For this review, take the finished solid that the model builds, in its own axes (mm). Face numbers are marked on the shaded views. A direction names the side the tool comes from. Give positions to 0.01 mm unless a question says otherwise; leave off trailing zeros. Order: outer loops, then holes, each group sorted by start corner. A loop starts at its lowest first (then second) coordinate and runs counter-clockwise, first axis right, second up. Notation, with made-up numbers: M 7,46 L 17,46 A9 cw 17,54 Z; hole C 1,69 d5. An arc over 180 degrees is marked long. Answer as CSV lines item,"result". Start each with the question number.
1. Clearance check with flat-ended pins moving along their axes: P1, Ø4, axis at x = -19.69, z = 24.25, coming from the -Y side; P2, Ø5, axis at x = -19.5, z = 26, coming from the +Y side; P3, Ø4.5, axis at x = -19.69, z = 9.25, coming from the +Y side. State where each tip first meets the part, or that it passes through.
2. We need section C-C, the plane y = -9. Give the boundary of the cut face in (x, z), and give its area (3 significant figures).
3. Machinability: for the marked faces 1, 2 and 3, which of the approach directions +Z, -Z, +X, -X, +Y, -Y give a long, thin tool a straight path to every point of the face, cutting with its end or side? Answer none if there is none.
4. Mouldability with a two-part tool opening along Z and no side actions: class the marked faces 4, 5, 6 and 7 as pulls with the +Z half, pulls with the -Z half, needs draft (parallel to the pull), parting line crosses it, or undercut.
5. We need section B-B, the plane x = -3. Give the boundary of the cut face in (y, z), and give its area (3 significant figures).
6. We need section D-D, the plane z = 17. Give the boundary of the cut face in (x, y), and give its area (3 significant figures).
7. For line 1 along X through (y, z) = (15, 9.25); line 2 along X through (y, z) = (8, -24); line 3 along Y through (x, z) = (0, -1), list the stretches that pass through material, from the lowest coordinate up.
8. We need section A-A, the plane y = 6.5. Give the boundary of the cut face in (x, z), and give its area (3 significant figures).
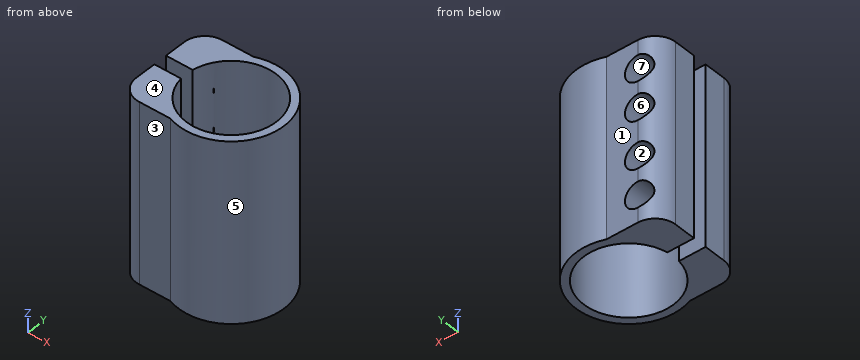
from build123d import *

# Parameters (mm, degrees)
F1_DEPTH       = 35
F3_D           = 5
F3_DEPTH       = 12
F3_START       = 1.7550021
F3_CBORE_D     = 10
F3_CBORE_DEPTH = 8
F3_TIP         = 1.5021515476


with BuildPart() as f1:
    # F0 (on Top) → F1 (new body, symmetric)
    with BuildSketch(Plane.XY):
        with BuildLine():
            ThreePointArc((-17.2933548246, 2.6813949562), (17.5, 0), (-17.2933548246, -2.6813949562))
            Line((-17.2933548246, -2.6813949562), (-27.6933548246, -2.6813949562))
            Line((-27.6933548246, -2.6813949562), (-27.6933548246, -11.0813949562))
            ThreePointArc((-27.6933548246, -11.0813949562), (-25.3502090741, -16.7382492056), (-19.6933548246, -19.0813949562))
            Line((-19.6933548246, -19.0813949562), (-7.4933548246, -19.0813949562))
            ThreePointArc((-7.4933548246, -19.0813949562), (20.5, 0), (-7.4933548246, 19.0813949562))
            Line((-7.4933548246, 19.0813949562), (-19.6933548246, 19.0813949562))
            ThreePointArc((-19.6933548246, 19.0813949562), (-25.3502090741, 16.7382492056), (-27.6933548246, 11.0813949562))
            Line((-27.6933548246, 11.0813949562), (-27.6933548246, 2.6813949562))
            Line((-27.6933548246, 2.6813949562), (-17.2933548246, 2.6813949562))
        make_face()
    extrude(amount=F1_DEPTH, both=True)

    # F3
    # its depths count from where the whole tool has entered the part; down to there all is cleared
    with Locations(Plane(origin=(0, 19.0813949562, 0), x_dir=(-1, 0, 0), z_dir=(0, 1, 0)).offset(-F3_START)):
        with Locations((19.6933548246, 24.25), (19.6933548246, 9.25), (19.6933548246, -9.25), (19.6933548246, -24.25)):
            CounterBoreHole(F3_D / 2, F3_CBORE_D / 2, F3_CBORE_DEPTH, depth=F3_DEPTH)
            with Locations((0, 0, -(F3_DEPTH + F3_TIP / 2))):  # 118° drill point
                Cone(0, F3_D / 2, F3_TIP, mode=Mode.SUBTRACT)


solid = f1.part
Result set:
1,P1,"y = -19.08"
1,P2,"y = 9.33"
1,P3,"y = 5.18"
2,outline,"M -27.69,-35 L -15.01,-35 L -15.01,35 L -27.69,35 Z; M 15.01,-35 L 18.42,-35 L 18.42,35 L 15.01,35 Z"
2,area,"1,130 mm2"
3,face 1,"+Z, -Z, -X, +Y"
3,face 2,"+Y"
3,face 3,"+Z, -Z, -X, -Y"
4,face 4,"pulls with the +Z half"
4,face 5,"needs draft"
4,face 6,"undercut"
4,face 7,"undercut"
5,outline,"M -20.28,-35 L -17.24,-35 L -17.24,35 L -20.28,35 Z; M 17.24,-35 L 20.28,-35 L 20.28,35 L 17.24,35 Z"
5,area,"425 mm2"
6,outline,"M -27.69,-11.08 A8 ccw -19.69,-19.08 L -7.49,-19.08 A20.5 ccw long -7.49,19.08 L -19.69,19.08 A8 ccw -27.69,11.08 L -27.69,2.68 L -17.29,2.68 A17.5 cw long -17.29,-2.68 L -27.69,-2.68 Z"
6,area,"687 mm2"
7,line 1,"-26.67 to -24.69, -14.69 to -9.01, 9.01 to 13.97"
7,line 2,"-27.69 to -22.18, -17.21 to -15.56, 15.56 to 18.87"
7,line 3,"-20.5 to -17.5, 17.5 to 20.5"
8,outline,"M -27.69,-35 L -16.25,-35 L -16.25,35 L -27.69,35 Z; M 16.25,-35 L 19.44,-35 L 19.44,35 L 16.25,35 Z; hole C -19.69,-24.25 d5; hole C -19.69,-9.25 d5; hole C -19.69,9.25 d5; hole C -19.69,24.25 d5"
8,area,"946 mm2"
